```python
from build123d import *

# Parameters (mm, degrees)
SKETCH_1_W          = 99.3
SKETCH_1_H          = 96.6
SKETCH_1_R          = 1.585
EXTRUDE_1_DEPTH     = 1.5
SKETCH_2_R          = 3.5
SKETCH_2_R_2        = 4
SKETCH_2_W          = 18.4
SKETCH_2_H          = 23.2
SKETCH_2_W_2        = 18
SKETCH_2_H_2        = 7.3
SKETCH_2_W_3        = 6.1
SKETCH_2_H_3        = 88.4
SKETCH_2_H_4        = 87.9
SKETCH_2_W_4        = 6.9
SKETCH_2_H_5        = 7.9
SKETCH_2_W_5        = 11
SKETCH_2_H_6        = 11.1
CUT_EXTRUDE_1_DEPTH = 117.077839401
SKETCH_3_W          = 1
SKETCH_3_H          = 2
EXTRUDE_2_DEPTH     = 1.5
CHAMFER_1_SIZE      = 1


with BuildPart() as part:
    # 草图1 → 凸台-拉伸1 (new body)
    with BuildSketch(Plane.XY):
        with Locations((31.77, 34.42)):
            Rectangle(SKETCH_1_W, SKETCH_1_H)
        with Locations((48.92, 64.16)):
            Circle(SKETCH_1_R, mode=Mode.SUBTRACT)
        with Locations((4.42, 64.16)):
            Circle(SKETCH_1_R, mode=Mode.SUBTRACT)
        with Locations((4.42, 4.42)):
            Circle(SKETCH_1_R, mode=Mode.SUBTRACT)
        with Locations((48.92, 4.42)):
            Circle(SKETCH_1_R, mode=Mode.SUBTRACT)
        with Locations((-9.08, 2.42)):
            Circle(SKETCH_1_R, mode=Mode.SUBTRACT)
        with Locations((72.92, -9.58)):
            Circle(SKETCH_1_R, mode=Mode.SUBTRACT)
        with Locations((72.92, 78.42)):
            Circle(SKETCH_1_R, mode=Mode.SUBTRACT)
        with Locations((-9.58, 79.42)):
            Circle(SKETCH_1_R, mode=Mode.SUBTRACT)
    extrude(amount=EXTRUDE_1_DEPTH)

    # 草图2 → 切除-拉伸1 (cut, through all)
    with BuildSketch(Plane.XY.offset(1.5)):
        with Locations((38.82, 58.16)):
            Circle(SKETCH_2_R)
        with Locations((-6.08, -8.08)):
            Circle(SKETCH_2_R_2)
        with Locations((61.52, 71.12)):
            Rectangle(SKETCH_2_W, SKETCH_2_H)
        with Locations((32.62, 46.11)):
            Rectangle(SKETCH_2_W_2, SKETCH_2_H_2)
        with Locations((-14.83, 34.62)):
            Rectangle(SKETCH_2_W_3, SKETCH_2_H_3)
        with Locations((78.37, 34.87)):
            Rectangle(SKETCH_2_W_3, SKETCH_2_H_4)
        with Locations((33.97, 11.07)):
            Rectangle(SKETCH_2_W_4, SKETCH_2_H_5)
        with Locations((-0.98, 77.17)):
            Rectangle(SKETCH_2_W_5, SKETCH_2_H_6)
    extrude(amount=-CUT_EXTRUDE_1_DEPTH, mode=Mode.SUBTRACT)

    # 草图3 → 凸台-拉伸2 (add)
    with BuildSketch(Plane.XY.offset(1.5)):
        with Locations((75.82, 77.82)):
            Rectangle(SKETCH_3_W, SKETCH_3_H)
    extrude(amount=-EXTRUDE_2_DEPTH)

    # 倒角1
    chamfer_1_edges = [part.edges().sort_by_distance(p)[0] for p in [
        (75.32, 76.82, 0.75),
    ]]
    chamfer(chamfer_1_edges, length=CHAMFER_1_SIZE - 0.0001)  # a hair under: the kernel refuses the full size


solid = part.part
```
Geometry: final body of the model. Coordinates: model frame, mm. Give positions to 0.01 mm unless a question says otherwise; leave off trailing zeros. Write each loop counter-clockwise with the first axis right and the second up, starting at its lowest first coordinate (ties: lowest second). Pieces come first, ordered by that corner, then holes.
1. Section query C-C, the plane x = 38.82. Return loops of the section in (y, z), then the cut area to 3 significant figures.
2. Section query B-B, the plane x = 48.92. Return loops of the section in (y, z) (3 decimals), then the cut area to 3 significant figures.
3. Line query: probe 1 along Y at (x, z) = (4.42, 0.4) (3 decimals); probe 2 along Y at (x, z) = (38.82, 0.8); probe 3 along X at (y, z) = (48.5, 1.3). Output: solid intervals per line, ascending.
4. Pin query (flat end, axial travel): P1, Ø0.8, axis at y = 77.5, z = 0.5, coming from the +X side; P2, Ø5, axis at x = 72.92, y = 78.42, coming from the -Z side. Return the tip coordinate at first contact, or that it passes through.
5. Section query A-A, the plane y = 69. Return loops of the section in (x, z), then the cut area to 3 significant figures.
6. Section query D-D, the plane z = 0.85. Count the separate pieces of the cut face and the enclosed holes in it, then the cut area to 3 significant figures.
7. Draft query along Y for faces 1 (the flat face through (31, 35, 1.5)), 2 (the cylindrical face through (72.71, -8.01, 0.74)). Return one class per face: released by +Y, released by -Y, zero draft, split by the parting line, or undercut.
Computed:
1. outline: (-13.88, 0) - (42.46, 0) - (42.46, 1.5) - (-13.88, 1.5) - close; (49.76, 0) - (54.66, 0) - (54.66, 1.5) - (49.76, 1.5) - close; (61.66, 0) - (82.72, 0) - (82.72, 1.5) - (61.66, 1.5) - close
1. area: 123 mm2
2. outline: (-13.88, 0) - (2.835, 0) - (2.835, 1.5) - (-13.88, 1.5) - close; (6.005, 0) - (62.575, 0) - (62.575, 1.5) - (6.005, 1.5) - close; (65.745, 0) - (82.72, 0) - (82.72, 1.5) - (65.745, 1.5) - close
2. area: 135 mm2
3. probe 1: y = -13.88 to 2.835, 6.005 to 62.575, 65.745 to 71.62
3. probe 2: y = -13.88 to 42.46, 49.76 to 54.66, 61.66 to 82.72
3. probe 3: x = -11.78 to 23.62, 41.62 to 75.32
4. P1: stops at x = 76.32
4. P2: stops at z = 0
5. outline: (-11.78, 0) - (52.32, 0) - (52.32, 1.5) - (-11.78, 1.5) - close; (70.72, 0) - (75.32, 0) - (75.32, 1.5) - (70.72, 1.5) - close
5. area: 103 mm2
6. separate pieces: 1
6. enclosed holes: 12
6. area: 7,630 mm2
7. face 1: zero draft
7. face 2: undercut
